from build123d import *

# Parameters (mm, degrees)
SKETCH1_W            = 20
SKETCH1_H            = 16
BOSS_EXTRUDE1_DEPTH  = 4
M3_CLEARANCE_HOLE1_D = 3.4
SKETCH4_W            = 27.686396546
SKETCH4_H            = 6.2
CUT_EXTRUDE1_DEPTH   = 2.3
FILLET1_R            = 1.5


with BuildPart() as part:
    # Sketch1 → Boss-Extrude1 (new body)
    with BuildSketch(Plane.XY):
        with Locations((10, 8)):
            Rectangle(SKETCH1_W, SKETCH1_H)
        with BuildLine():
            Line((6.5, 11.1), (6.5, 4.9))
            ThreePointArc((6.5, 4.9), (5, 3.4), (3.5, 4.9))
            Line((3.5, 4.9), (3.5, 11.1))
            ThreePointArc((3.5, 11.1), (5, 12.6), (6.5, 11.1))
        make_face(mode=Mode.SUBTRACT)
    extrude(amount=BOSS_EXTRUDE1_DEPTH)

    # M3 Clearance Hole1 (through all)
    with Locations(Plane.XY.offset(4)):
        with Locations((13.25, 13.5), (13.25, 2.5)):
            Hole(M3_CLEARANCE_HOLE1_D / 2)

    # Sketch4 → Cut-Extrude1 (cut)
    with BuildSketch(Plane.XY.offset(4)):
        with Locations((12.569554471, 8)):
            Rectangle(SKETCH4_W, SKETCH4_H)
    extrude(amount=-CUT_EXTRUDE1_DEPTH, mode=Mode.SUBTRACT)

    # Fillet1
    fillet1_edges = [part.edges().sort_by_distance(p)[0] for p in [
        (20, 8, 1.7),
    ]]
    fillet(fillet1_edges, radius=FILLET1_R)


solid = part.part
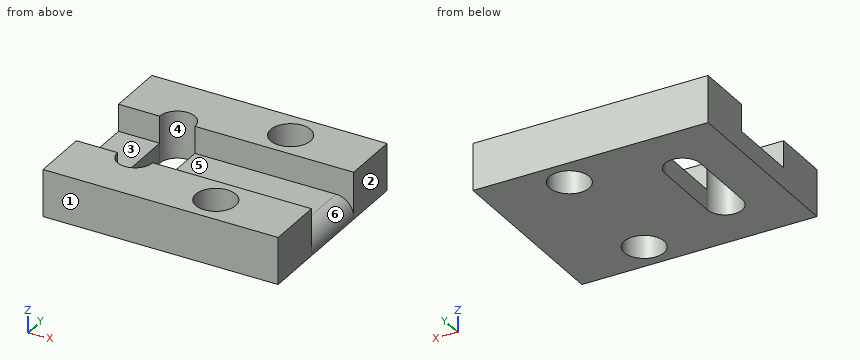
Could you check a few things on this model? Use its own coordinates, in mm. Face numbers are marked on the shaded views. A direction names the side the tool comes from. Give positions to 0.01 mm unless a question says otherwise; leave off trailing zeros. Write each loop counter-clockwise with the first axis right and the second up, starting at its lowest first coordinate (ties: lowest second). Pieces come first, ordered by that corner, then holes. Notation, with made-up numbers: (12.5, 68) -> (17.5, 68) arc R9 ccw to (17.5, 85) -> close; hole circle Ø2 at (74, 8). An arc over 180 degrees is marked (long way). Answer as a JSON object with one key per item and string values.
Q1. Suppose I cut it at B-B on z = 3.25. Write out the boundary of the cut face in (x, y), then the cut area to 3 significant figures.
Taken from the geometry:
{"outline": "(0, 0) -> (20, 0) -> (20, 4.9) -> (6.5, 4.9) arc R1.5 cw to (3.5, 4.9) -> (0, 4.9) -> close; (0, 11.1) -> (3.5, 11.1) arc R1.5 cw to (6.5, 11.1) -> (20, 11.1) -> (20, 16) -> (0, 16) -> close; hole circle Ø3.4 at (13.25, 2.5); hole circle Ø3.4 at (13.25, 13.5)", "area": "171 mm²"}
Q2. Will these pins go through, and if not, where does the flat tip stop? pin 1 Ø2 at (x, y) = (13.25, 13.5) entering from +Z; pin 2 Ø3 at (x, y) = (1, 9.5) entering from +Z; pin 3 Ø0.8 at (y, z) = (8.5, 1) entering from +X.
Taken from the geometry:
{"pin 1": "passes through", "pin 2": "stops at z = 1.7", "pin 3": "stops at x = 19.95"}
Q3. Suppose I cut it at A-A on x = 13.25. Write out the boundary of the cut face in (y, z).
Taken from the geometry:
{"outline": "(0, 0) -> (0.8, 0) -> (0.8, 4) -> (0, 4) -> close; (4.2, 0) -> (11.8, 0) -> (11.8, 4) -> (11.1, 4) -> (11.1, 1.7) -> (4.9, 1.7) -> (4.9, 4) -> (4.2, 4) -> close; (15.2, 0) -> (16, 0) -> (16, 4) -> (15.2, 4) -> close"}
Q4. Suppose I cut it at C-C on y = 13.5. Write out the boundary of the cut face in (x, z), then the cut area to 3 significant figures.
Taken from the geometry:
{"outline": "(0, 0) -> (11.55, 0) -> (11.55, 4) -> (0, 4) -> close; (14.95, 0) -> (20, 0) -> (20, 4) -> (14.95, 4) -> close", "area": "66.4 mm²"}
Q5. Which directions (+Z, -Z, +X, -X, +Y, -Y) give clear straight access to the entire face, cutting with the end or side of a thin tool? Please do the marked faces 4, 5 and 6.
Taken from the geometry:
{"face 4": "+Z, -Z", "face 5": "+Z, +X, -X", "face 6": "+Z, +X"}
Q6. Suppose I cut it at D-D on x = 5. Write out the boundary of the cut face in (y, z), then the cut area to 3 significant figures.
Taken from the geometry:
{"outline": "(0, 0) -> (3.4, 0) -> (3.4, 4) -> (0, 4) -> close; (12.6, 0) -> (16, 0) -> (16, 4) -> (12.6, 4) -> close", "area": "27.2 mm²"}
Q7. Please list where these lines run through material, in increasing order: L1, parallel to Y at x = 13.25, z = 0.9; L2, parallel to Y at x = 13.25, z = 3; L3, parallel to Y at x = 18.5, z = 3.55.
Taken from the geometry:
{"L1": "y = 0 to 0.8, 4.2 to 11.8, 15.2 to 16", "L2": "y = 0 to 0.8, 4.2 to 4.9, 11.1 to 11.8, 15.2 to 16", "L3": "y = 0 to 4.9, 11.1 to 16"}
Q8. We'd pull the mould along Y, two halves only. Please class the marked faces 1, 2 and 3: released by +Y, released by -Y, zero draft, split by the parting line, or undercut.
Taken from the geometry:
{"face 1": "released by -Y", "face 2": "zero draft", "face 3": "undercut"}
